Geometry check sheet. Reference: the model listing, model coordinates, mm. Face numbers are marked on the shaded views. A direction names the side the tool comes from. Round coordinates to 2 decimals unless told otherwise and drop trailing zeros. Loops run counter-clockwise (first coordinate to the right, second up) from the corner with the lowest first, then second, coordinate; pieces in that order, holes last. Notation, with made-up numbers: M 34.25,-11 L 43.25,-11 A25 cw 43.25,10 Z; hole C 7.25,25.25 d2. An arc over 180 degrees is marked long. Answer in a Markdown table with one row per item. Add a question column.
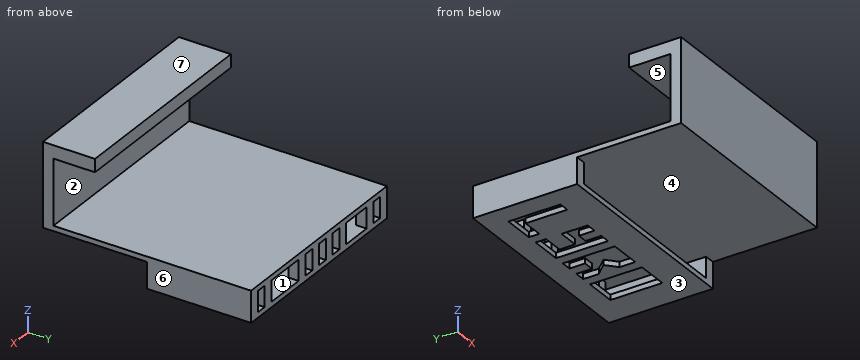
```python
from build123d import *

# Parameters (mm, degrees)
F0_W     = 4
F0_H     = 2
F0_H_2   = 8
F1_DEPTH = 40
F2_DEPTH = 80
F4_DEPTH = 80
F5_DEPTH = 4
F6_W     = 12
F6_H     = 20
F7_DEPTH = 25


with BuildPart() as f1:
    # F0 (on Front) → F1 (new body)
    with BuildSketch(Plane.XZ):
        with Locations((-78, -11)):
            Rectangle(F0_W, F0_H)
        with Locations((-74, -11)):
            Rectangle(F0_W, F0_H)
        with Locations((-70, -11)):
            Rectangle(F0_W, F0_H)
        with Locations((-66, -11)):
            Rectangle(F0_W, F0_H)
        with Locations((-62, -11)):
            Rectangle(F0_W, F0_H)
        with Locations((-58, -11)):
            Rectangle(F0_W, F0_H)
        with Locations((-54, -11)):
            Rectangle(F0_W, F0_H)
        with Locations((-50, -11)):
            Rectangle(F0_W, F0_H)
        with Locations((-46, -11)):
            Rectangle(F0_W, F0_H)
        with Locations((-42, -11)):
            Rectangle(F0_W, F0_H)
        with Locations((-38, -11)):
            Rectangle(F0_W, F0_H)
        with Locations((-34, -11)):
            Rectangle(F0_W, F0_H)
        with Locations((-30, -11)):
            Rectangle(F0_W, F0_H)
        with Locations((-26, -11)):
            Rectangle(F0_W, F0_H)
        with Locations((-22, -11)):
            Rectangle(F0_W, F0_H)
        with Locations((-18, -11)):
            Rectangle(F0_W, F0_H)
        with Locations((-14, -11)):
            Rectangle(F0_W, F0_H)
        with Locations((-10, -11)):
            Rectangle(F0_W, F0_H)
        with Locations((-6, -11)):
            Rectangle(F0_W, F0_H)
        with Locations((-2, -11)):
            Rectangle(F0_W, F0_H)
        with Locations((-78, -6)):
            Rectangle(F0_W, F0_H_2)
        with Locations((-2, -6)):
            Rectangle(F0_W, F0_H_2)
    extrude(amount=F1_DEPTH)

    # F0 (on Front) → F2 (join)
    with BuildSketch(Plane.XZ):
        with Locations((-78, -1)):
            Rectangle(F0_W, F0_H)
        with Locations((-70, -1)):
            Rectangle(F0_W, F0_H)
        with Locations((-74, -1)):
            Rectangle(F0_W, F0_H)
        with Locations((-66, -1)):
            Rectangle(F0_W, F0_H)
        with Locations((-62, -1)):
            Rectangle(F0_W, F0_H)
        with Locations((-58, -1)):
            Rectangle(F0_W, F0_H)
        with Locations((-54, -1)):
            Rectangle(F0_W, F0_H)
        with Locations((-50, -1)):
            Rectangle(F0_W, F0_H)
        with Locations((-46, -1)):
            Rectangle(F0_W, F0_H)
        with Locations((-42, -1)):
            Rectangle(F0_W, F0_H)
        with Locations((-38, -1)):
            Rectangle(F0_W, F0_H)
        with Locations((-34, -1)):
            Rectangle(F0_W, F0_H)
        with Locations((-30, -1)):
            Rectangle(F0_W, F0_H)
        with Locations((-26, -1)):
            Rectangle(F0_W, F0_H)
        with Locations((-22, -1)):
            Rectangle(F0_W, F0_H)
        with Locations((-18, -1)):
            Rectangle(F0_W, F0_H)
        with Locations((-14, -1)):
            Rectangle(F0_W, F0_H)
        with Locations((-6, -1)):
            Rectangle(F0_W, F0_H)
        with Locations((-2, -1)):
            Rectangle(F0_W, F0_H)
        with Locations((-10, -1)):
            Rectangle(F0_W, F0_H)
    extrude(amount=F2_DEPTH)

    # F3 (on Right) → F4 (join)
    with BuildSketch(Plane.YZ):
        Polygon((-80, 30), (-80, 0), (-76, 0), (-76, 25), (-60, 25), (-60, 30), align=None)
    extrude(amount=-F4_DEPTH)

    # F0 (on Front) → F5 (join)
    with BuildSketch(Plane.XZ):
        with Locations((-70, -6)):
            Rectangle(F0_W, F0_H_2)
        with Locations((-54, -6)):
            Rectangle(F0_W, F0_H_2)
        with Locations((-46, -6)):
            Rectangle(F0_W, F0_H_2)
        with Locations((-38, -6)):
            Rectangle(F0_W, F0_H_2)
        with Locations((-30, -6)):
            Rectangle(F0_W, F0_H_2)
        with Locations((-10, -6)):
            Rectangle(F0_W, F0_H_2)
    extrude(amount=F5_DEPTH)

    # F6 (on face) → F7 (cut)
    with BuildSketch(Plane(origin=(0, 0, -2), x_dir=(1, 0, 0), z_dir=(0, 0, -1))):
        Polygon((-68, 28.3951728637), (-72, 28.3951728637), (-72, 8.3951728637), (-60, 8.3951728637), (-60, 12.3951728637), (-68, 12.3951728637), align=None)
        with Locations((-18, 18.3951728637)):
            Rectangle(F6_W, F6_H)
        Polygon((-52, 28.3951728637), (-56, 28.3951728637), (-56, 18.3951728637), (-48, 18.3951728637), (-48, 12.3951728637), (-56, 12.3951728637), (-56, 8.3951728637), (-44, 8.3951728637), (-44, 28.3951728637), (-48, 28.3951728637), (-48, 22.3951728637), (-52, 22.3951728637), align=None)
        Polygon((-28, 28.3951728637), (-40, 28.3951728637), (-40, 8.3951728637), (-36, 8.3951728637), (-36.0326175784, 14.3950842042), (-32, 14.3950842042), (-32, 8.3951728637), (-28, 8.3951728637), (-28, 14.3951728637), (-31.9809810322, 18.7847752528), (-28, 22.3951728637), align=None)
    extrude(amount=F7_DEPTH, mode=Mode.SUBTRACT)


solid = f1.part
```
1) Thickness scan on L1, parallel to X at y = -12.5, z = -7.5; L2, parallel to Z at x = -10.5, y = -9.5; L3, parallel to Z at x = -7.5, y = -75. Record the ranges inside material, lowest first. Write a range as [from, to].
2) Cross-section at A-A, the plane x = -58. Record the boundary of the cut face in (y, z), plus the area to 3 significant figures.
3) Go/stop test with flat-tipped pins: pin 1 (4 mm diameter, centred on x = -16.5, z = 15.5, fed in from +Y); pin 2 (8 mm diameter, centred on x = -61.5, y = -19, fed in from +Z); pin 3 (4.5 mm diameter, centred on x = -30, z = -8, fed in from -Y). Record where each tip stops, or that it passes through.
4) Cross-section at D-D, the plane y = -6. Record the boundary of the cut face in (x, z).
5) Cross-section at B-B, the plane y = -70.5. Record the boundary of the cut face in (x, z), plus the area to 3 significant figures.
6) Cross-section at C-C, the plane x = -67. Record the boundary of the cut face in (y, z).
7) Set-up check for the marked faces 1, 2 and 3: record each of +Z, -Z, +X, -X, +Y, -Y from which the full face is reachable in a straight line by a thin tool's end or side.
8) Draft check along Z on the marked faces 4, 5, 6 and 7. Enter one of: +Z half, -Z half, draft (parallel to the pull), parting line (faces both ways), or undercut.
Worked answers:
| question | item | result |
|---|---|---|
| 1 | L1 | x = [-80, -76], [-4, 0] |
| 1 | L2 | z = [-12, -10], [-2, 0] |
| 1 | L3 | z = [-2, 0], [25, 30] |
| 2 | outline | M -80,-2 L 0,-2 L 0,0 L -76,0 L -76,25 L -60,25 L -60,30 L -80,30 Z; M -40,-12 L 0,-12 L 0,-10 L -40,-10 Z |
| 2 | area | 440 mm2 |
| 3 | pin 1 | stops at y = -76 |
| 3 | pin 2 | stops at z = 0 |
| 3 | pin 3 | stops at y = -40 |
| 4 | outline | M -80,-12 L 0,-12 L 0,0 L -80,0 Z; hole M -76,-10 L -4,-10 L -4,-2 L -76,-2 Z |
| 5 | outline | M -80,-2 L 0,-2 L 0,0 L -80,0 Z; M -80,25 L 0,25 L 0,30 L -80,30 Z |
| 5 | area | 560 mm2 |
| 6 | outline | M -80,-2 L 0,-2 L 0,0 L -76,0 L -76,25 L -60,25 L -60,30 L -80,30 Z; M -40,-12 L -12.4,-12 L -12.4,-10 L -40,-10 Z; M -8.4,-12 L 0,-12 L 0,-10 L -8.4,-10 Z |
| 7 | face 1 | -Y |
| 7 | face 2 | +X, -X, +Y |
| 7 | face 3 | -Z, +X, -X, +Y, -Y |
| 8 | face 4 | undercut |
| 8 | face 5 | undercut |
| 8 | face 6 | draft |
| 8 | face 7 | +Z half |
